```python
from build123d import *

# Parameters (mm, degrees)
PAD_DEPTH = 90


with BuildPart() as part:
    # Sketch → Pad (new body)
    with BuildSketch(Plane.XZ):
        Polygon((-39.462553, 5.478498), (-39.4624, -9.521502), (62.033083, -9.521502), (62.033083, 3.99388), (-14.042966, 3.99388), (1.486176, 61.94943), (-3.843011, 63.434039), (-19.372154, 5.478489), (-19.385466, -4.521511), (-34.101345, -4.521511), (-34.101345, 5.478498), align=None)
    extrude(amount=PAD_DEPTH)


solid = part.part
```
Build history of the part. All positions in model axes, mm. A direction names the side the tool comes from. Give positions to 0.01 mm unless a question says otherwise; leave off trailing zeros. Loops run counter-clockwise (first coordinate to the right, second up) from the corner with the lowest first, then second, coordinate; pieces in that order, holes last. Notation, with made-up numbers: (-26.75, 88.5) - (10.25, 88.5) arc R22 ccw to (10.25, 113.5) - close; hole circle Ø1 at (10.25, 52.5). An arc over 180 degrees is marked (long way). Use a Markdown table: item, result.
(1) Band-saw the part on D-D (z = 50). Give the cut face in (x, y), and give its area (3 significant figures).
Taken from the geometry:
| item | result |
|---|---|
| outline | (-7.44, -90) - (-1.72, -90) - (-1.72, 0) - (-7.44, 0) - close |
| area | 515 mm2 |
(2) Wall check: line 1 along X through (y, z) = (-45.5, -2); line 2 along Z through (x, y) = (52, -30); line 3 along Z through (x, y) = (-35, -78). Give the ranges that are in metal, low to high.
Taken from the geometry:
| item | result |
|---|---|
| line 1 | -39.46 to -34.1, -19.38 to 62.03 |
| line 2 | -9.52 to 3.99 |
| line 3 | -9.52 to 5.48 |
(3) Band-saw the part on B-B (x = -8.5). Give the cut face in (y, z).
Taken from the geometry:
| item | result |
|---|---|
| outline | (-90, -9.52) - (0, -9.52) - (0, 3.99) - (-90, 3.99) - close; (-90, 24.68) - (0, 24.68) - (0, 46.05) - (-90, 46.05) - close |
(4) Pull direction X, two halves, no side cores. Call faces 1 (the face through (-11.5, -44.37, 34.86)), 2 (the face through (-34.101, -44, 0)), 3 (the face through (11, 0, 3)): +X half, -X half, draft (parallel to the pull), parting line (faces both ways), or undercut.
Taken from the geometry:
| item | result |
|---|---|
| face 1 | -X half |
| face 2 | undercut |
| face 3 | draft |
(5) Drop flat-ended pins along their axis: pin 1 Ø6 at (x, y) = (9, -67) entering from +Z; pin 2 Ø1.6 at (x, y) = (-37, -42) entering from +Z; pin 3 Ø4.5 at (x, y) = (-28, -30.5) entering from +Z. Give the stop position or say it passes through.
Taken from the geometry:
| item | result |
|---|---|
| pin 1 | z = 3.99 |
| pin 2 | z = 5.48 |
| pin 3 | z = -4.52 |
(6) Which spindle directions (+Z, -Z, +X, -X, +Y, -Y) get a long thin tool onto all of the face, cutting with end or side? Do faces 4 (the face through (-27, -44, -4.522)), 5 (the face through (-37, -44, 5.478)), 6 (the face through (-6.387, -44.37, 32.566)). Say none if no direction does.
Taken from the geometry:
| item | result |
|---|---|
| face 4 | +Z, +Y, -Y |
| face 5 | +Z, -X, +Y, -Y |
| face 6 | +X, +Y, -Y |
(7) Band-saw the part on A-A (y = -66.5). Give the cut face in (x, z).
Taken from the geometry:
| item | result |
|---|---|
| outline | (-39.46, -9.52) - (62.03, -9.52) - (62.03, 3.99) - (-14.04, 3.99) - (1.49, 61.95) - (-3.84, 63.43) - (-19.37, 5.48) - (-19.39, -4.52) - (-34.1, -4.52) - (-34.1, 5.48) - (-39.46, 5.48) - close |
(8) Band-saw the part on C-C (x = 3). Give the cut face in (y, z).
Taken from the geometry:
| item | result |
|---|---|
| outline | (-90, -9.52) - (0, -9.52) - (0, 3.99) - (-90, 3.99) - close |
